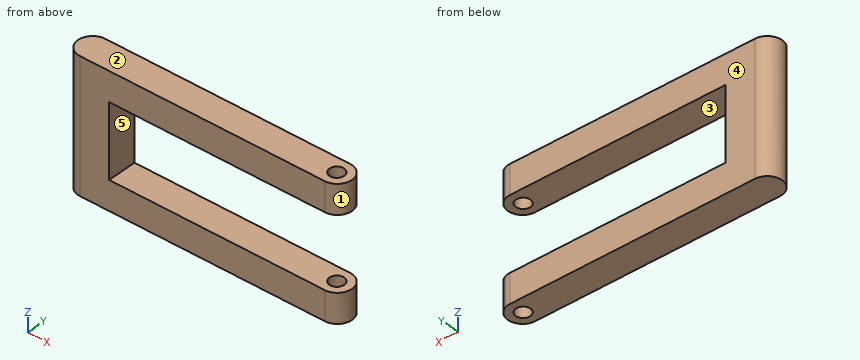
```python
from build123d import *

# Parameters (mm, degrees)
BOSS_EXTRUDE1_DEPTH = 4
BOSS_EXTRUDE2_DEPTH = 10
BOSS_EXTRUDE3_DEPTH = 4
SKETCH4_R           = 1
CUT_EXTRUDE4_DEPTH  = 26


with BuildPart() as part:
    # Sketch1 → Boss-Extrude1 (new body)
    with BuildSketch(Plane.XY):
        with BuildLine():
            Line((0, 0), (33.5, 0))
            ThreePointArc((33.5, 0), (35.5, 2), (33.5, 4))
            Line((33.5, 4), (0, 4))
            ThreePointArc((0, 4), (-2, 2), (0, 0))
        make_face()
    extrude(amount=BOSS_EXTRUDE1_DEPTH)

    # Sketch2 → Boss-Extrude2 (add)
    with BuildSketch(Plane.XY.offset(4)):
        with BuildLine():
            Line((4, 0), (0, 0))
            ThreePointArc((0, 0), (-2, 2), (0, 4))
            Line((0, 4), (4, 4))
            Line((4, 4), (4, 0))
        make_face()
    extrude(amount=BOSS_EXTRUDE2_DEPTH)

    # Sketch3 → Boss-Extrude3 (add)
    with BuildSketch(Plane.XY.offset(14)):
        with BuildLine():
            Line((0, 4), (33.5, 4))
            ThreePointArc((33.5, 4), (35.5, 2), (33.5, 0))
            Line((33.5, 0), (0, 0))
            ThreePointArc((0, 0), (-2, 2), (0, 4))
        make_face()
    extrude(amount=BOSS_EXTRUDE3_DEPTH)

    # Sketch4 → Cut-Extrude4 (cut)
    with BuildSketch(Plane.XY.offset(18)):
        with Locations((33.427257806, 2)):
            Circle(SKETCH4_R)
    extrude(amount=-CUT_EXTRUDE4_DEPTH, mode=Mode.SUBTRACT)


solid = part.part
```
Check sheet for the modelled part. Datum: model origin and axes. Units: mm. Face numbers are marked on the shaded views. A direction names the side the tool comes from. Round coordinates to 2 decimals unless told otherwise and drop trailing zeros. Order: outer loops, then holes, each group sorted by start corner. A loop starts at its lowest first (then second) coordinate and runs counter-clockwise, first axis right, second up. Notation, with made-up numbers: M -5.5,67 L 30.5,67 A17 cw 30.5,76 Z; hole C 27.25,-31 d10. An arc over 180 degrees is marked long. Answer in a Markdown table with one row per item.
(1) Section check B-B on y = 2. Record the boundary of the cut face in (x, z), plus the area to 3 significant figures.
Findings:
| item | result |
|---|---|
| outline | M -2,0 L 32.43,0 L 32.43,4 L 4,4 L 4,14 L 32.43,14 L 32.43,18 L -2,18 Z; M 34.43,0 L 35.5,0 L 35.5,4 L 34.43,4 Z; M 34.43,14 L 35.5,14 L 35.5,18 L 34.43,18 Z |
| area | 344 mm^2 |
(2) Gauge pin test, flat end, axial feed: pin 1 (1.5 mm diameter, centred on y = 2.5, z = 5, fed in from +X). Record the tip position at first contact, or that the pin passes through.
Findings:
| item | result |
|---|---|
| pin 1 | stops at x = 4 |
(3) Material ranges on line 1 along Z through (x, y) = (12, 1.6); line 2 along X through (y, z) = (1.1, 17); line 3 along X through (y, z) = (3.15, 5.75), recorded low to high. Write a range as from..to.
Findings:
| item | result |
|---|---|
| line 1 | z = 0..4, 14..18 |
| line 2 | x = -1.79..32.99, 33.86..35.29 |
| line 3 | x = -1.64..4 |
(4) Section check C-C on z = 10.25. Record the boundary of the cut face in (x, y), plus the area to 3 significant figures.
Findings:
| item | result |
|---|---|
| outline | M 0,0 L 4,0 L 4,4 L 0,4 A2 ccw Z |
| area | 22.3 mm^2 |
(5) Draft check along Z on the marked faces 1, 2 and 3. Enter one of: +Z half, -Z half, draft (parallel to the pull), parting line (faces both ways), or undercut.
Findings:
| item | result |
|---|---|
| face 1 | draft |
| face 2 | +Z half |
| face 3 | undercut |
(6) Section check A-A on x = 12. Record the boundary of the cut face in (y, z).
Findings:
| item | result |
|---|---|
| outline | M 0,0 L 4,0 L 4,4 L 0,4 Z; M 0,14 L 4,14 L 4,18 L 0,18 Z |
(7) Set-up check for the marked faces 4 and 5: record each of +Z, -Z, +X, -X, +Y, -Y from which the full face is reachable in a straight line by a thin tool's end or side.
Findings:
| item | result |
|---|---|
| face 4 | +Z, -Z, +X, -X, +Y |
| face 5 | +X, +Y, -Y |
